The model under review builds one solid part; all positions refer to its coordinate system, in mm. Face numbers are marked on the shaded views. A direction names the side the tool comes from. Round coordinates to 2 decimals unless told otherwise and drop trailing zeros. Write each loop counter-clockwise with the first axis right and the second up, starting at its lowest first coordinate (ties: lowest second). Pieces come first, ordered by that corner, then holes. Notation, with made-up numbers: M 71,25.5 L 96,25.5 A34 ccw 96,61.5 Z; hole C 87,47 d6. An arc over 180 degrees is marked long. Write item = value, one per line. Start each with the question number.
Item 1: The part is to be moulded in two halves that separate along Y. For the marked faces 1, 2 and 3, say which applies: +Y half, -Y half, draft (parallel to the pull), parting line (faces both ways), or undercut.
Item 2: To check wall thickness, follow line 1 along Y through (x, z) = (20, 15); line 2 along Z through (x, y) = (17.5, 5); line 3 along X through (y, z) = (1, 23). State the ranges of each line that lie inside material, in increasing order.
Item 3: Take a section at B-B, the plane x = -4. Give the boundary of the cut face in (y, z), plus the area to 3 significant figures.
Item 4: Take a section at D-D, the plane x = -14. Give the boundary of the cut face in (y, z).
Item 5: For pin 1 Ø3 at (y, z) = (11, 25.5) entering from -X; pin 2 Ø6 at (x, z) = (-35, 12.5) entering from +Y; pin 3 Ø12 at (y, z) = (16.5, 11.5) entering from +X; pin 4 Ø11 at (y, z) = (5, 15) entering from +X, all flat-tipped, find the tip position at first contact; note any pin that passes through.
Item 6: Tool access review of the marked faces 4, 5 and 6: name each direction out of +Z, -Z, +X, -X, +Y, -Y from which nothing blocks a thin tool from reaching the whole face with its end or side.
Item 7: Take a section at C-C, the plane y = 1. Give the boundary of the cut face in (x, z), plus the area to 3 significant figures.
Item 8: Take a section at A-A, the plane z = 28. Give the boundary of the cut face in (x, y).
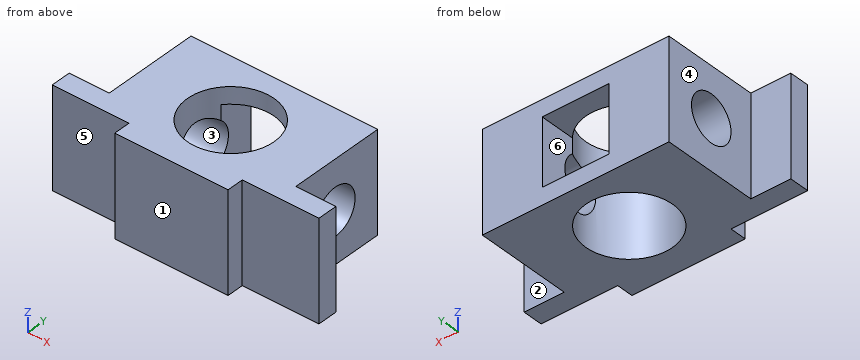
from build123d import *

# Parameters (mm, degrees)
EXTRUDE_1_DEPTH     = 30
SKETCH_2_R          = 13
CUT_EXTRUDE_1_DEPTH = 54.851648071
SKETCH_3_R          = 7
CUT_EXTRUDE_2_DEPTH = 77.96752562
CUT_EXTRUDE_3_REACH = 66.031
SKETCH_4_W          = 20
SKETCH_4_H          = 20


with BuildPart() as part:
    # Эскиз1 → Бобышка-Вытянуть1 (new body)
    with BuildSketch(Plane.XY):
        Polygon((-40, -15), (-17, -15), (-17, -20), (17, -20), (17, -15), (40, -15), (40, -9), (28, -9), (28, 20), (-28, 20), (-28, -9), (-40, -9), align=None)
    extrude(amount=EXTRUDE_1_DEPTH)

    # Эскиз2 → Вырез-Вытянуть1 (cut, through all)
    with BuildSketch(Plane.XY.offset(30)):
        with Locations((0, 1)):
            Circle(SKETCH_2_R)
    extrude(amount=-CUT_EXTRUDE_1_DEPTH, mode=Mode.SUBTRACT)

    # Эскиз3 → Вырез-Вытянуть2 (cut, through all)
    with BuildSketch(Plane.ZY.offset(28)):
        with Locations((15, 5)):
            Circle(SKETCH_3_R)
    extrude(amount=-CUT_EXTRUDE_2_DEPTH, mode=Mode.SUBTRACT)

    # Эскиз4 → Вырез-Вытянуть3 (cut, up to next)
    with BuildSketch(Plane(origin=(0, 20, 0), x_dir=(1, 0, 0), z_dir=(0, 1, 0)), mode=Mode.PRIVATE) as cut_extrude_3_sk1:
        with Locations((0, -15)):
            Rectangle(SKETCH_4_W, SKETCH_4_H)
    cut_extrude_3_tool1 = extrude(cut_extrude_3_sk1.sketch, amount=-CUT_EXTRUDE_3_REACH, mode=Mode.PRIVATE) & part.part
    add(cut_extrude_3_tool1.solids().sort_by_distance((0, 20, 15))[0], mode=Mode.SUBTRACT)


solid = part.part
Response values:
q1.face_1 = -Y half
q1.face_2 = +Y half
q1.face_3 = undercut
q2.line_1 = -15 to -2, 12 to 20
q2.line_2 = 0 to 8, 22 to 30
q2.line_3 = -28 to -13, 13 to 28
q3.outline = M -20,0 L -11.37,0 L -11.37,30 L -20,30 Z; M 13.37,0 L 20,0 L 20,5 L 13.37,5 Z; M 13.37,25 L 20,25 L 20,30 L 13.37,30 Z
q3.area = 325 mm2
q4.outline = M -20,0 L 20,0 L 20,30 L -20,30 Z; hole C 5,15 d14
q5.pin_1 = -28
q5.pin_2 = -9
q5.pin_3 = 28
q5.pin_4 = through
q6.face_4 = +Z, -Z, -X, +Y
q6.face_5 = +Z, -Z, -X, -Y
q6.face_6 = +Y
q7.outline = M -28,0 L -13,0 L -13,9.26 L -28,9.26 Z; M -28,20.74 L -13,20.74 L -13,30 L -28,30 Z; M 13,0 L 28,0 L 28,9.26 L 13,9.26 Z; M 13,20.74 L 28,20.74 L 28,30 L 13,30 Z
q7.area = 555 mm2
q8.outline = M -40,-15 L -17,-15 L -17,-20 L 17,-20 L 17,-15 L 40,-15 L 40,-9 L 28,-9 L 28,20 L -28,20 L -28,-9 L -40,-9 Z; hole C 0,1 d26
